Geometry check sheet. Reference: the model listing, model coordinates, mm. Coordinates: 2 decimals unless noted, no trailing zeros. Order: outer loops, then holes, each group sorted by start corner. A loop starts at its lowest first (then second) coordinate and runs counter-clockwise, first axis right, second up. Notation, with made-up numbers: (38, 85.5) - (62, 85.5) arc R21 ccw to (62, 113.5) - close; hole circle Ø9 at (58, 59.5). An arc over 180 degrees is marked (long way). Put each result on its own line as item: value.
Autodesk Inventor part; units mm, degrees
ref_plane "YZ Plane" through (0, 0, 0) normal (1, 0, 0) x (0, 1, 0)
ref_plane "XZ Plane" through (0, 0, 0) normal (0, 1, 0) x (-1, 0, 0)
ref_plane "XY Plane" through (0, 0, 0) normal (0, 0, 1) x (1, 0, 0)
sketch "Sketch1" plane through (0, 0, 0) normal (0, 1, 0) x (-1, 0, 0)
  line L0 (55, -26.5) -> (-55, -26.5)
  line L1 (-55, -26.5) -> (-55, 26.5)
  line L2 (-55, 26.5) -> (55, 26.5)
  line L3 (55, 26.5) -> (55, -26.5)
  point P0 (0, 0)
  point P1 (0, -26.5)
  point P2 (55, 0)
  dimension "d0" = 53
  dimension "d1" = 110
extrude "Extrusion1" add sketch "Sketch1" along normal blind 1.6
sketch "Sketch2" plane through (0, 1.6, 0) normal (0, 1, 0) x (1, 0, 0)
  line L0 (55, 26.5) -> (-55, 26.5)
  line L1 (-55, 26.5) -> (-55, -26.5)
  line L2 (-55, -26.5) -> (55, -26.5)
  line L3 (55, -26.5) -> (55, 26.5)
  point P0 (0, 0)
  point P1 (-48, -19.5)
  point P2 (-48, 19.5)
  point P3 (48, -19.5)
  point P4 (48, 19.5)
  dimension "d4" = 7
  dimension "d5" = 7
  dimension "d6" = 7
  dimension "d7" = 7
hole "Hole1" at (-48, 1.6, 19.5) at (-48, 1.6, -19.5) at (48, 1.6, 19.5) at (48, 1.6, -19.5) direction (0, -1, 0) diameter 3 end through all
properties part number "Heater_pcb"
Q1. Draft check along X on faces 1 (the cylindrical face through (-46.536, 0.789, 19.175)), 2 (the flat face through (1, 0, 0)). Enter one of: pulls with the +X half, pulls with the -X half, needs draft (parallel to the pull), parting line crosses it, or undercut.
Answer block:
face 1: undercut
face 2: needs draft
Q2. Section check A-A on z = -19.5. Record the boundary of the cut face in (x, y).
Answer block:
outline: (-55, 0) - (-49.5, 0) - (-49.5, 1.6) - (-55, 1.6) - close; (-46.5, 0) - (46.5, 0) - (46.5, 1.6) - (-46.5, 1.6) - close; (49.5, 0) - (55, 0) - (55, 1.6) - (49.5, 1.6) - close
Q3. Depth check by flat-ended pin: pin 1 Ø1.8 at (x, z) = (48, -19.5) entering from +Y. Enter the tip coordinate at first touch or a pass-through.
Answer block:
pin 1: passes through
Q4. Section check B-B on x = -48. Record the boundary of the cut face in (y, z), then the cut area to 3 significant figures.
Answer block:
outline: (0, -26.5) - (1.6, -26.5) - (1.6, -21) - (0, -21) - close; (0, -18) - (1.6, -18) - (1.6, 18) - (0, 18) - close; (0, 21) - (1.6, 21) - (1.6, 26.5) - (0, 26.5) - close
area: 75.2 mm^2
Q5. Thickness scan on L1, parallel to X at y = 0.55, z = -19.5; L2, parallel to Z at x = 48, y = 1.15; L3, parallel to X at y = 1.45, z = 18.5. Record the ranges inside material, lowest first. Write a range as [from, to].
Answer block:
L1: x = [-55, -49.5], [-46.5, 46.5], [49.5, 55]
L2: z = [-26.5, -21], [-18, 18], [21, 26.5]
L3: x = [-55, -49.12], [-46.88, 46.88], [49.12, 55]
